Read the model definition and answer for the solid it produces. Units are mm, in the model's axes. Coordinates: 2 decimals unless noted, no trailing zeros. Write each loop counter-clockwise with the first axis right and the second up, starting at its lowest first coordinate (ties: lowest second). Pieces come first, ordered by that corner, then holes.
Item 1: Section B-B (y = 12.7) is taken. Give the vertices of the cut face in (x, z), then the cut area to 3 significant figures.
Item 2: Determine the mould class of faces 1 (the face through (-50.555, -13.803, 0.783)), 2 (the face through (-1, 0, 0)) for opening direction X: released by +X, released by -X, zero draft, split by the parting line, or undercut.
Item 3: Straight lines are drawn through the part: probe 1 along Y at (x, z) = (-25.4, 0.4); probe 2 along X at (y, z) = (13.5, 0.45); probe 3 along Y at (x, z) = (50, 1.45). For each, find the intervals that lie inside material, in ascending order.
Item 4: Section A-A (x = 25.4) is taken. Give the vertices of the cut face in (y, z), then the cut area to 3 significant figures.
from build123d import *

# Parameters (mm, degrees)
SKETCH1_W             = 124.3
SKETCH1_H             = 35.4
BOSS_EXTRUDE1_DEPTH   = 1.5875
F_4_40_TAPPED_HOLE1_D = 2.2606
LPATTERN1_COUNT       = 5
LPATTERN1_PITCH       = 25.4


with BuildPart() as part:
    # Sketch1 → Boss-Extrude1 (new body)
    with BuildSketch(Plane.XY):
        Rectangle(SKETCH1_W, SKETCH1_H)
    extrude(amount=BOSS_EXTRUDE1_DEPTH)

    # #4-40 Tapped Hole1 (through all)
    with Locations(Plane(origin=(-50.8, 12.7, 1.5875), x_dir=(1, 0, 0), z_dir=(0, 0, 1))):
        with Locations((0, 0), (0, -25.4)):
            f_4_40_tapped_hole1 = Hole(F_4_40_TAPPED_HOLE1_D / 2)

    # LPattern1: #4-40 Tapped Hole1 ×5
    with Locations(*[(i * LPATTERN1_PITCH, 0, 0) for i in range(1, LPATTERN1_COUNT)]):
        add(f_4_40_tapped_hole1, mode=Mode.SUBTRACT)


solid = part.part
Established:
1. outline: (-62.15, 0) - (-51.93, 0) - (-51.93, 1.59) - (-62.15, 1.59) - close; (-49.67, 0) - (-26.53, 0) - (-26.53, 1.59) - (-49.67, 1.59) - close; (-24.27, 0) - (-1.13, 0) - (-1.13, 1.59) - (-24.27, 1.59) - close; (1.13, 0) - (24.27, 0) - (24.27, 1.59) - (1.13, 1.59) - close; (26.53, 0) - (49.67, 0) - (49.67, 1.59) - (26.53, 1.59) - close; (51.93, 0) - (62.15, 0) - (62.15, 1.59) - (51.93, 1.59) - close
1. area: 179 mm2
2. face 1: undercut
2. face 2: zero draft
3. probe 1: y = -17.7 to -13.83, -11.57 to 11.57, 13.83 to 17.7
3. probe 2: x = -62.15 to -51.6, -50 to -26.2, -24.6 to -0.8, 0.8 to 24.6, 26.2 to 50, 51.6 to 62.15
3. probe 3: y = -17.7 to -13.5, -11.9 to 11.9, 13.5 to 17.7
4. outline: (-17.7, 0) - (-13.83, 0) - (-13.83, 1.59) - (-17.7, 1.59) - close; (-11.57, 0) - (11.57, 0) - (11.57, 1.59) - (-11.57, 1.59) - close; (13.83, 0) - (17.7, 0) - (17.7, 1.59) - (13.83, 1.59) - close
4. area: 49.0 mm2
